Build history of the part. All positions in model axes, mm. A direction names the side the tool comes from. Give positions to 0.01 mm unless a question says otherwise; leave off trailing zeros. Order: outer loops, then holes, each group sorted by start corner. A loop starts at its lowest first (then second) coordinate and runs counter-clockwise, first axis right, second up. Notation, with made-up numbers: (-29, -27) - (-6, -27) arc R23 cw to (-6, -16) - close; hole circle Ø1 at (-5, 2). An arc over 180 degrees is marked (long way). Answer in a Markdown table with one row per item.
```python
from build123d import *

# Parameters (mm, degrees)
F1_DEPTH  = 15
F5_DEPTH  = 23
F6_DEPTH  = 19
F2_R      = 3.5
F7_DEPTH  = 25
F8_DEPTH  = 2.5
F12_DEPTH = 19
F13_DEPTH = 23
F14_DEPTH = 2.5
F15_DEPTH = 25
F17_DEPTH = 25


with BuildPart() as f1:
    # F0 (on Front) → F1 (new body)
    with BuildSketch(Plane.XZ):
        Polygon((47.5, 0), (36, 5), (36, 2.5), (36, 0), align=None)
        Polygon((-36, -20), (-36, -5), (-59, -5), (-59, -20.0883084536), align=None)
        Polygon((-36, -5), (-36, 0), (-47.5, 0), (-59, 0), (-59, -5), align=None)
        Polygon((-36, 0), (-36, 5), (-47.5, 0), align=None)
        Polygon((36, 5), (-36, 5), (-36, 0), (-36, -5), (36, -5), (36, 0), (36, 2.5), align=None)
        Polygon((59, 0), (47.5, 0), (36, 0), (36, -5), (36, -20), (59, -20.0883084536), (59, -5), align=None)
    extrude(amount=F1_DEPTH)

    # F3 (on face) → F5 (cut)
    with BuildSketch(Plane.YZ.offset(59)):
        with BuildLine():
            ThreePointArc((-5.75, -13.0883084536), (-8.7374368671, -11.8508715865), (-7.5, -14.8383084536))
            ThreePointArc((-7.5, -14.8383084536), (-6.2625631329, -14.3257453206), (-5.75, -13.0883084536))
        make_face()
    extrude(amount=-F5_DEPTH, mode=Mode.SUBTRACT)

    # F3 (on face) → F6 (cut)
    with BuildSketch(Plane.YZ.offset(59)):
        with BuildLine():
            ThreePointArc((-4.5, -13.0883084536), (-9.6213203436, -10.96698811), (-7.5, -16.0883084536))
            ThreePointArc((-7.5, -16.0883084536), (-5.3786796564, -15.2096287971), (-4.5, -13.0883084536))
        make_face()
        with BuildLine():
            ThreePointArc((-5.75, -13.0883084536), (-6.2625631329, -14.3257453206), (-7.5, -14.8383084536))
            ThreePointArc((-7.5, -14.8383084536), (-8.7374368671, -11.8508715865), (-5.75, -13.0883084536))
        make_face(mode=Mode.SUBTRACT)
    extrude(amount=-F6_DEPTH, mode=Mode.SUBTRACT)

    # F2 (on face) → F7 (cut)
    with BuildSketch(Plane(origin=(-0.0762581326, 0, -19.8614852797), x_dir=(0.9999926292, 0, -0.0038394697), z_dir=(-0.0038394697, 0, -0.9999926292))):
        with Locations((54.0766935746, 7.5)):
            Circle(F2_R)
    extrude(amount=-F7_DEPTH, mode=Mode.SUBTRACT)

    # F4 (on face) → F8 (cut)
    with BuildSketch(Plane(origin=(36, 0, 0), x_dir=(0, -1, 0), z_dir=(-1, 0, 0))):
        Polygon((4.675, -15.825), (7.5, -15.825), (10.325, -15.825), (10.325, -10.175), (4.675, -10.175), align=None)
    extrude(amount=-F8_DEPTH, mode=Mode.SUBTRACT)

    # F9 (on face) → F12 (cut)
    with BuildSketch(Plane(origin=(-59, 0, 0), x_dir=(0, -1, 0), z_dir=(-1, 0, 0))):
        with BuildLine():
            ThreePointArc((10.5, -13.0883084536), (5.3786796564, -10.96698811), (7.5, -16.0883084536))
            ThreePointArc((7.5, -16.0883084536), (9.6213203436, -15.2096287971), (10.5, -13.0883084536))
        make_face()
        with BuildLine():
            ThreePointArc((9.25, -13.0883084536), (8.7374368671, -14.3257453206), (7.5, -14.8383084536))
            ThreePointArc((7.5, -14.8383084536), (6.2625631329, -11.8508715865), (9.25, -13.0883084536))
        make_face(mode=Mode.SUBTRACT)
    extrude(amount=-F12_DEPTH, mode=Mode.SUBTRACT)

    # F9 (on face) → F13 (cut)
    with BuildSketch(Plane(origin=(-59, 0, 0), x_dir=(0, -1, 0), z_dir=(-1, 0, 0))):
        with BuildLine():
            ThreePointArc((9.25, -13.0883084536), (6.2625631329, -11.8508715865), (7.5, -14.8383084536))
            ThreePointArc((7.5, -14.8383084536), (8.7374368671, -14.3257453206), (9.25, -13.0883084536))
        make_face()
    extrude(amount=-F13_DEPTH, mode=Mode.SUBTRACT)

    # F10 (on face) → F14 (cut)
    with BuildSketch(Plane.YZ.offset(-36)):
        Polygon((-10.325, -15.825), (-7.5, -15.825), (-4.675, -15.825), (-4.675, -10.175), (-10.325, -10.175), align=None)
    extrude(amount=-F14_DEPTH, mode=Mode.SUBTRACT)

    # F11 (on face) → F15 (cut)
    with BuildSketch(Plane(origin=(0.0762581326, 0, -19.8614852797), x_dir=(0.9999926292, 0, 0.0038394697), z_dir=(0.0038394697, 0, -0.9999926292))):
        with BuildLine():
            ThreePointArc((-50.5766935746, 7.5), (-54.0766935746, 11), (-57.5766935746, 7.5))
            ThreePointArc((-57.5766935746, 7.5), (-54.0766935746, 4), (-50.5766935746, 7.5))
        make_face()
    extrude(amount=-F15_DEPTH, mode=Mode.SUBTRACT)

    # F16 (on face) → F17 (cut)
    with BuildSketch(Plane.XY.offset(5)):
        with BuildLine():
            ThreePointArc((-13.8871266544, -7.5), (-17.8871266544, -3.5), (-21.8871266544, -7.5))
            Line((-21.8871266544, -7.5), (-13.8871266544, -7.5))
        make_face()
        with BuildLine():
            ThreePointArc((21.8871266544, -7.5), (17.8871266544, -3.5), (13.8871266544, -7.5))
            Line((13.8871266544, -7.5), (21.8871266544, -7.5))
        make_face()
        with BuildLine():
            Line((21.8871266544, -7.5), (13.8871266544, -7.5))
            ThreePointArc((13.8871266544, -7.5), (17.8871266544, -11.5), (21.8871266544, -7.5))
        make_face()
        with BuildLine():
            ThreePointArc((4, -7.5), (0, -3.5), (-4, -7.5))
            Line((-4, -7.5), (4, -7.5))
        make_face()
        with BuildLine():
            Line((4, -7.5), (-4, -7.5))
            ThreePointArc((-4, -7.5), (0, -11.5), (4, -7.5))
        make_face()
        with BuildLine():
            Line((-13.8871266544, -7.5), (-21.8871266544, -7.5))
            ThreePointArc((-21.8871266544, -7.5), (-17.8871266544, -11.5), (-13.8871266544, -7.5))
        make_face()
    extrude(amount=-F17_DEPTH, mode=Mode.SUBTRACT)


solid = f1.part
```
1. Cut at A-A on x = 0. Write the cut outline in (y, z).
Check result:
| item | result |
|---|---|
| outline | (-15, -5) - (-11.5, -5) - (-11.5, 5) - (-15, 5) - close; (-3.5, -5) - (0, -5) - (0, 5) - (-3.5, 5) - close |
2. Cut at C-C on z = -18.5. Count the separate pieces of the cut face and the enclosed holes in it, and give its area (3 significant figures).
Check result:
| item | result |
|---|---|
| separate pieces | 2 |
| enclosed holes | 2 |
| area | 613 mm² |
3. Drop flat-ended pins along their axis: P1, Ø3, axis at x = -37.5, y = -8, coming from the -Z side; P2, Ø3, axis at y = -8, z = -14, coming from the +X side; P3, Ø7, axis at x = 0, y = -7.5, coming from the -Z side; P4, Ø7.5, axis at x = -17, y = -5, coming from the -Z side. Give the stop position or say it passes through.
Check result:
| item | result |
|---|---|
| P1 | stops at z = -20.01 |
| P2 | stops at x = 40 |
| P3 | passes through |
| P4 | stops at z = -5 |
4. Cut at D-D on x = 15. Write the cut outline in (y, z).
Check result:
| item | result |
|---|---|
| outline | (-15, -5) - (-10.27, -5) - (-10.27, 5) - (-15, 5) - close; (-4.73, -5) - (0, -5) - (0, 5) - (-4.73, 5) - close |
5. Which spindle directions (+Z, -Z, +X, -X, +Y, -Y) get a long thin tool onto all of the face, cutting with end or side? Do faces 1 (the face through (37, -7, -15.825)), 2 (the face through (-50.6, -5.7, 0)), 3 (the face through (-1, -12, -5)), 4 (the face through (50.8, -5.7, 0)). Say none if no direction does.
Check result:
| item | result |
|---|---|
| face 1 | none |
| face 2 | +Z, -X, +Y, -Y |
| face 3 | -Z, +Y, -Y |
| face 4 | +Z, +X, +Y, -Y |
6. Probe line 1 (X direction, y = -1.25, z = -12.5); line 2 (X direction, y = -10, z = 1); line 3 (X direction, y = -5.5, z = 3.25) (3 decimals). List the from-to ranges inside material, lowest first.
Check result:
| item | result |
|---|---|
| line 1 | x = -59 to -36, 36 to 59 |
| line 2 | x = -45.2 to -21.01, -14.76 to -3.12, 3.12 to 14.76, 21.01 to 45.2 |
| line 3 | x = -40.025 to -21.351, -14.423 to -3.464, 3.464 to 14.423, 21.351 to 40.025 |
7. Two-plate mould, pull along X, no slides. Class faces 5 (the face through (-59, -7.4, -9.9)), 6 (the face through (-38.5, -8.8, -11.7)), 7 (the face through (40, -8, -15)): +X half, -X half, draft (parallel to the pull), parting line (faces both ways), or undercut.
Check result:
| item | result |
|---|---|
| face 5 | -X half |
| face 6 | undercut |
| face 7 | +X half |
8. Cut at B-B on y = -12.5. Write the cut outline in (x, z).
Check result:
| item | result |
|---|---|
| outline | (-59, -20.09) - (-36, -20) - (-36, -5) - (36, -5) - (36, -20) - (59, -20.09) - (59, 0) - (47.5, 0) - (36, 5) - (-36, 5) - (-47.5, 0) - (-59, 0) - close |
